Input: part model. Units: mm. Frame: model coordinates. A direction names the side the tool comes from. Coordinates: 2 decimals unless noted, no trailing zeros. Order: outer loops, then holes, each group sorted by start corner. A loop starts at its lowest first (then second) coordinate and runs counter-clockwise, first axis right, second up. Notation, with made-up numbers: M 15.25,0 L 64.25,0 A25 ccw 64.25,23 Z; hole C -36,-6 d2. An arc over 180 degrees is marked long. Answer in a Markdown table with one row per item.
from build123d import *

# Parameters (mm, degrees)
SKETCH012_R     = 1.9
PAD005_DEPTH    = 9.6
SKETCH013_R     = 1.025
PAD006_DEPTH    = 2
CHAMFER002_SIZE = 0.4
CHAMFER003_SIZE = 0.4


with BuildPart() as part:
    # Sketch012 → Pad005 (new body)
    with BuildSketch(Plane.XY):
        Circle(SKETCH012_R)
    extrude(amount=PAD005_DEPTH)

    # Sketch013 (on Face3 of Pad005) → Pad006 (join)
    with BuildSketch(Plane.XY.offset(9.6)):
        Circle(SKETCH013_R)
    extrude(amount=PAD006_DEPTH)

    # Chamfer002
    chamfer002_edges = [part.edges().sort_by_distance(p)[0] for p in [
        (-1.025, 0, 11.6),
    ]]
    chamfer(chamfer002_edges, length=CHAMFER002_SIZE)

    # Chamfer003
    chamfer003_edges = [part.edges().sort_by_distance(p)[0] for p in [
        (-1.9, 0, 9.6),
    ]]
    chamfer(chamfer003_edges, length=CHAMFER003_SIZE)


with BuildPart() as part_1:
    # Body002 placement: moved
    add(part.part.moved(Location((27.1, 44.5, 0))))


solid = part_1.part
1) Cut plane B-B, the plane x = 27.1. Output: boundary loops of the cut face in (y, z) (3 decimals), and give its area (3 significant figures).
Resolved:
| item | result |
|---|---|
| outline | M 42.6,0 L 46.4,0 L 46.4,9.2 L 46,9.6 L 45.525,9.6 L 45.525,11.2 L 45.125,11.6 L 43.875,11.6 L 43.475,11.2 L 43.475,9.6 L 43,9.6 L 42.6,9.2 Z |
| area | 40.3 mm2 |
2) Material intervals for probe 1 along X at (y, z) = (46.1, 7.5); probe 2 along Z at (x, y) = (28.1, 43.8); probe 3 along Y at (x, z) = (28.1, 1.5), sorted ascending.
Resolved:
| item | result |
|---|---|
| probe 1 | x = 26.08 to 28.12 |
| probe 2 | z = 0 to 9.6 |
| probe 3 | y = 42.88 to 46.12 |
3) Cut plane A-A, the plane y = 44.5. Output: boundary loops of the cut face in (x, z) (3 decimals).
Resolved:
| item | result |
|---|---|
| outline | M 25.2,0 L 29,0 L 29,9.2 L 28.6,9.6 L 28.125,9.6 L 28.125,11.2 L 27.725,11.6 L 26.475,11.6 L 26.075,11.2 L 26.075,9.6 L 25.6,9.6 L 25.2,9.2 Z |
4) Contact query for a flat-ended pin moving along its axis: pin 1 (1.5 mm diameter, centred on x = 28.5, z = 7, fed in from +Y). Output: stop coordinate, or through.
Resolved:
| item | result |
|---|---|
| pin 1 | stops at y = 46.29 |
5) Reachability of faces 1 (the face through (26.967, 45.516, 10.389)), 2 (the face through (27.1, 44.5, 11.6)) from +Z, -Z, +X, -X, +Y, -Y: full face, straight path, thin tool, end or side. Return the list, or none.
Resolved:
| item | result |
|---|---|
| face 1 | +Z |
| face 2 | +Z, +X, -X, +Y, -Y |
6) Cut plane C-C, the plane z = 0.5. Output: boundary loops of the cut face in (x, y), and give its area (3 significant figures).
Resolved:
| item | result |
|---|---|
| outline | C 27.1,44.5 d3.8 |
| area | 11.3 mm2 |
7) Cut plane D-D, the plane z = 10.5. Output: boundary loops of the cut face in (x, y) (3 decimals).
Resolved:
| item | result |
|---|---|
| outline | C 27.1,44.5 d2.05 |
